Can you work these out from the model? Positions are in its coordinate system, mm. A direction names the side the tool comes from. Coordinates: 2 decimals unless noted, no trailing zeros. Write each loop counter-clockwise with the first axis right and the second up, starting at its lowest first coordinate (ties: lowest second). Pieces come first, ordered by that corner, then holes. Notation, with made-up numbers: (35, 86) - (42, 86) arc R22 cw to (42, 119) - close; hole circle Ø4 at (-16.75, 20). An arc over 180 degrees is marked (long way). Use one line per item in the form item = value. Start each with the question number.
(1) If we section it at D-D on y = 19.5: Please give me the cut outline in (x, z), then the cut area to 3 significant figures.
(2) For pin 1 Ø1 at (x, z) = (-15.5, 6.5) entering from +Y; pin 2 Ø10 at (x, y) = (-4, 7.5) entering from +Z; pin 3 Ø7.5 at (x, z) = (-14, 44.5) entering from -Y; pin 4 Ø3.5 at (x, z) = (-5, 44.25) entering from -Y, each with a flat end and sliding along its axis, tell me the tip position at first contact or that it passes through.
(3) Thinking about a two-plate mould opening in Z: for faces 6 (the face through (-10, 13, 0)), 7 (the face through (-12.854, 28.268, -4.426)), 8 (the face through (-10, 0, 21)), which applies, pulls with the +Z half, pulls with the -Z half, needs draft (parallel to the pull), parting line crosses it, or undercut?
(4) If I drill on probe 1 along X at (y, z) = (28.05, -3.75); probe 2 along Z at (x, y) = (-5, 28.6); probe 3 along Y at (x, z) = (-7.5, 27), over which ranges is the centre line in solid material (lowest first)? Write a range as from..to.
(5) If we section it at A-A on z = 44.25: Please give me the cut outline in (x, y).
(6) On a 3-axis mill with a long thin cutter (end or side, diameter ignored), from which of +Z, -Z, +X, -X, +Y, -Y can I reach the whole of each face in a straight line? I mean faces 1 (the face through (-10, 29.5, 44)), 2 (the face through (-10, 34, 0)), 3 (the face through (-10, 27, -3)), 4 (the face through (-10, 14, 40.5)), 5 (the face through (-12.4, 40, 8.7)). Say none if no direction works.
(7) If we section it at B-B on x = -15: Please give me the cut outline in (y, z).
(8) If we section it at C-C on x = -10: Please give me the cut outline in (y, z), then the cut area to 3 significant figures.
Autodesk Inventor part; units mm, degrees
ref_plane "YZ Plane" through (0, 0, 0) normal (1, 0, 0) x (0, 1, 0)
ref_plane "XZ Plane" through (0, 0, 0) normal (0, 1, 0) x (-1, 0, 0)
ref_plane "XY Plane" through (0, 0, 0) normal (0, 0, 1) x (1, 0, 0)
sketch "Sketch1" plane through (0, 0, 0) normal (1, 0, 0) x (0, 1, 0)
  line L0 (38, 40.5) -> (0, 40.5)
  line L1 (0, 40.5) -> (0, 0)
  line L2 (0, 0) -> (38, 0)
  line L3 (38, 0) -> (38, 40.5)
  dimension "d0" = 40.5
  dimension "d1" = 38
extrude "BODY" add sketch "Sketch1" against normal blind 20
sketch "Sketch2" plane through (0, 0, 40.5) normal (0, 0, 1) x (1, 0, 0)
  line L0 (-20, 0) -> (-20, 38) construction
  line L1 (0, 0) -> (-20, 0) construction
  line L2 (0, 27) -> (-20, 27)
  line L3 (-20, 27) -> (-20, 29.5)
  line L4 (-20, 29.5) -> (0, 29.5)
  line L5 (0, 29.5) -> (0, 27)
  dimension "d4" = 27
  dimension "d5" = 2.5
  dimension "d6" = 20
  dimension "d7" = 0
extrude "BRACKET1" add sketch "Sketch2" along normal blind 6.85
sketch "Sketch3" plane through (0, 0, 0) normal (0, 0, -1) x (-1, 0, 0)
  line L0 (0, 0) -> (0, 38) construction
  line L1 (0, 0) -> (20, 0) construction
  line L2 (20, 27) -> (0, 27)
  line L3 (0, 27) -> (0, 29.5)
  line L4 (0, 29.5) -> (20, 29.5)
  line L5 (20, 29.5) -> (20, 27)
  dimension "d10" = 27
  dimension "d11" = 2.5
  dimension "d12" = 0
  dimension "d13" = 20
extrude "BRACKET2" add sketch "Sketch3" along normal blind 6.85
sketch "Sketch4" plane through (-20, 29.5, 40.5) normal (0, 1, 0) x (1, 0, 0)
  line L0 (0, 0) -> (20, 0) construction
  line L1 (20, 0) -> (20, -6.85) construction
  circle A0 centre (5, -3.75) radius 2.25
  circle A1 centre (15, -3.75) radius 2.25
  circle A2 centre (5, 44.25) radius 2.25
  circle A3 centre (15, 44.25) radius 2.25
  line L2 (20, 40.5) -> (20, 47.35) construction
  line L3 (0, 40.5) -> (0, 47.35) construction
  dimension "d16" = 4.5
  dimension "d17" = 4.5
  dimension "d18" = 4.5
  dimension "d19" = 4.5
  dimension "d20" = 48
  dimension "d21" = 48
  dimension "d22" = 10
  dimension "d23" = 5
  dimension "d24" = 5
  dimension "d26" = 10
  dimension "d27" = 3.75
  dimension "d28" = 5
extrude "SCREW_HOLES" cut sketch "Sketch4" against normal blind 10
sketch "Sketch5" plane through (0, 38, 40.5) normal (0, 1, 0) x (1, 0, 0)
  line L0 (-20, 0) -> (-20, 40.5) construction
  line L1 (0, 0) -> (-20, 0) construction
  circle A0 centre (-10, 30) radius 3
  dimension "d31" = 6
  dimension "d32" = 30
  dimension "d33" = 10
extrude "TORQUE_CENTER" add sketch "Sketch5" along normal blind 4
equation "\"d10\" = d4"
equation "\"d11\" = d5"
equation "\"d13\" = d6"
equation "\"d14\" = d8"
equation "\"d17\" = d16"
equation "\"d18\" = d16"
equation "\"d19\" = d16"
properties part number "JX PDI-HV5932MG-180 digital servo" material "JX PDI-HV5932MG-180 digital servo color"
Reported:
q1.outline = (-20, 0) - (0, 0) - (0, 40.5) - (-20, 40.5) - close
q1.area = 810 mm2
q2.pin_1 = 38
q2.pin_2 = 40.5
q2.pin_3 = 27
q2.pin_4 = through
q3.face_6 = pulls with the -Z half
q3.face_7 = undercut
q3.face_8 = needs draft
q4.probe_1 = -20..-17.25, -12.75..-7.25, -2.75..0
q4.probe_2 = -6.85..-6, -1.5..42, 46.5..47.35
q4.probe_3 = 0..38
q5.outline = (-20, 27) - (-17.25, 27) - (-17.25, 29.5) - (-20, 29.5) - close; (-12.75, 27) - (-7.25, 27) - (-7.25, 29.5) - (-12.75, 29.5) - close; (-2.75, 27) - (0, 27) - (0, 29.5) - (-2.75, 29.5) - close
q6.face_1 = +Z, +X, -X, +Y
q6.face_2 = -Z, +X, -X, +Y
q6.face_3 = -Z, +X, -X, -Y
q6.face_4 = +Z, +X, -X, -Y
q6.face_5 = +Y
q7.outline = (0, 0) - (27, 0) - (27, -1.5) - (29.5, -1.5) - (29.5, 0) - (38, 0) - (38, 40.5) - (29.5, 40.5) - (29.5, 42) - (27, 42) - (27, 40.5) - (0, 40.5) - close; (27, -6.85) - (29.5, -6.85) - (29.5, -6) - (27, -6) - close; (27, 46.5) - (29.5, 46.5) - (29.5, 47.35) - (27, 47.35) - close
q8.outline = (0, 0) - (27, 0) - (27, -6.85) - (29.5, -6.85) - (29.5, 0) - (38, 0) - (38, 7.5) - (42, 7.5) - (42, 13.5) - (38, 13.5) - (38, 40.5) - (29.5, 40.5) - (29.5, 47.35) - (27, 47.35) - (27, 40.5) - (0, 40.5) - close
q8.area = 1,600 mm2
